Geometry: final body of the model. Coordinates: model frame, mm. Round coordinates to 2 decimals unless told otherwise and drop trailing zeros. Loops run counter-clockwise (first coordinate to the right, second up) from the corner with the lowest first, then second, coordinate; pieces in that order, holes last. Notation, with made-up numbers: (72, 14) -> (131, 14) arc R17 cw to (131, 24) -> close; hole circle Ø2 at (85.25, 77). An arc over 180 degrees is marked (long way). Answer in a Markdown table with one row per item.
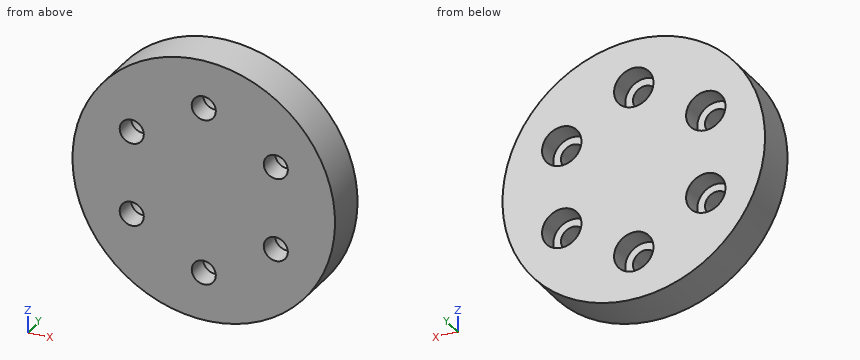
```python
from build123d import *

# Parameters (mm, degrees)
SKETCH1_R           = 30
BOSS_EXTRUDE1_DEPTH = 10
SKETCH2_R           = 4.5
CUT_EXTRUDE1_DEPTH  = 5
SKETCH3_R           = 2.75
CUT_EXTRUDE2_DEPTH  = 43.720018727


with BuildPart() as part:
    # Sketch1 → Boss-Extrude1 (new body)
    with BuildSketch(Plane(origin=(0, 0, 0), x_dir=(1, 0, 0), z_dir=(0, 1, 0))):
        with Locations(Location((0, 0, 0), (0, 0, 270))):
            Circle(SKETCH1_R)
    extrude(amount=BOSS_EXTRUDE1_DEPTH)

    # Sketch2 → Cut-Extrude1 (cut)
    with BuildSketch(Plane(origin=(0, 10, 0), x_dir=(1, 0, 0), z_dir=(0, 1, 0))):
        with Locations(Location((0, 19, 0), (0, 0, 270))):
            Circle(SKETCH2_R)
        with Locations(Location((16.454482672, 9.5, 0), (0, 0, 270))):
            Circle(SKETCH2_R)
        with Locations(Location((16.454482672, -9.5, 0), (0, 0, 270))):
            Circle(SKETCH2_R)
        with Locations(Location((0, -19, 0), (0, 0, 270))):
            Circle(SKETCH2_R)
        with Locations(Location((-16.454482672, -9.5, 0), (0, 0, 270))):
            Circle(SKETCH2_R)
        with Locations(Location((-16.454482672, 9.5, 0), (0, 0, 270))):
            Circle(SKETCH2_R)
    extrude(amount=-CUT_EXTRUDE1_DEPTH, mode=Mode.SUBTRACT)

    # Sketch3 → Cut-Extrude2 (cut, through all)
    with BuildSketch(Plane(origin=(0, 5, 0), x_dir=(1, 0, 0), z_dir=(0, 1, 0))):
        with Locations(Location((0, 19, 0), (0, 0, 270))):
            Circle(SKETCH3_R)
        with Locations(Location((16.454482672, 9.5, 0), (0, 0, 270))):
            Circle(SKETCH3_R)
        with Locations(Location((16.454482672, -9.5, 0), (0, 0, 270))):
            Circle(SKETCH3_R)
        with Locations(Location((0, -19, 0), (0, 0, 270))):
            Circle(SKETCH3_R)
        with Locations(Location((-16.454482672, -9.5, 0), (0, 0, 270))):
            Circle(SKETCH3_R)
        with Locations(Location((-16.454482672, 9.5, 0), (0, 0, 270))):
            Circle(SKETCH3_R)
    extrude(amount=-CUT_EXTRUDE2_DEPTH, mode=Mode.SUBTRACT)


solid = part.part
```
Item 1: Section query D-D, the plane z = 21. Output: boundary loops of the cut face in (x, y).
Ans:
| item | result |
|---|---|
| outline | (-21.42, 0) -> (-1.89, 0) -> (-1.89, 5) -> (-4.03, 5) -> (-4.03, 10) -> (-21.42, 10) -> close; (1.89, 0) -> (21.42, 0) -> (21.42, 10) -> (4.03, 10) -> (4.03, 5) -> (1.89, 5) -> close |
Item 2: Ray query, L1, parallel to Z at x = 4, y = 6.75; L2, parallel to Z at x = 12.5, y = 5.5; L3, parallel to X at y = 1.35, z = -9.5. Return the intervals inside material, ascending.
Ans:
| item | result |
|---|---|
| L1 | -29.73 to -21.06, -16.94 to 16.94, 21.06 to 29.73 |
| L2 | -27.27 to -11.65, -7.35 to 7.35, 11.65 to 27.27 |
| L3 | -28.46 to -19.2, -13.7 to 13.7, 19.2 to 28.46 |
Item 3: Section query A-A, the plane z = -9.5. Output: boundary loops of the cut face in (x, y).
Ans:
| item | result |
|---|---|
| outline | (-28.46, 0) -> (-19.2, 0) -> (-19.2, 5) -> (-20.95, 5) -> (-20.95, 10) -> (-28.46, 10) -> close; (-13.7, 0) -> (13.7, 0) -> (13.7, 5) -> (11.95, 5) -> (11.95, 10) -> (-11.95, 10) -> (-11.95, 5) -> (-13.7, 5) -> close; (19.2, 0) -> (28.46, 0) -> (28.46, 10) -> (20.95, 10) -> (20.95, 5) -> (19.2, 5) -> close |
Item 4: Section query C-C, the plane y = 5.75. Output: boundary loops of the cut face in (x, z).
Ans:
| item | result |
|---|---|
| outline | circle Ø60 at (0, 0); hole circle Ø9 at (-16.45, -9.5); hole circle Ø9 at (-16.45, 9.5); hole circle Ø9 at (0, -19); hole circle Ø9 at (0, 19); hole circle Ø9 at (16.45, -9.5); hole circle Ø9 at (16.45, 9.5) |
Item 5: Section query B-B, the plane x = 0. Output: boundary loops of the cut face in (y, z), and give its area (3 significant figures).
Ans:
| item | result |
|---|---|
| outline | (0, -30) -> (10, -30) -> (10, -23.5) -> (5, -23.5) -> (5, -21.75) -> (0, -21.75) -> close; (0, -16.25) -> (5, -16.25) -> (5, -14.5) -> (10, -14.5) -> (10, 14.5) -> (5, 14.5) -> (5, 16.25) -> (0, 16.25) -> close; (0, 21.75) -> (5, 21.75) -> (5, 23.5) -> (10, 23.5) -> (10, 30) -> (0, 30) -> close |
| area | 455 mm2 |
Item 6: First-contact query: P1, Ø8, axis at x = -16.45, z = -9.5, coming from the +Y side; P2, Ø3.5, axis at x = 16.45, z = -9.5, coming from the -Y side; P3, Ø5, axis at y = 5.5, z = -22, coming from the +X side; P4, Ø6, axis at y = 9, z = 16.5, coming from the +X side. Flat tips, straight axial feed; report the tip coordinate or a pass-through.
Ans:
| item | result |
|---|---|
| P1 | y = 5 |
| P2 | through |
| P3 | x = 22.8 |
| P4 | x = 26.79 |
